```python
from build123d import *

# Parameters (mm, degrees)
F0_R     = 2.5
F1_DEPTH = 3
F2_R     = 1.5
F3_DEPTH = 10
F4_R     = 2.286


with BuildPart() as f1:
    # F0 (on Front) → F1 (new body)
    with BuildSketch(Plane.XZ):
        Circle(F0_R)
    extrude(amount=F1_DEPTH)

    # F2 (on face) → F3 (join)
    with BuildSketch(Plane(origin=(0, 0, 0), x_dir=(-1, 0, 0), z_dir=(0, 1, 0))):
        Circle(F2_R)
    extrude(amount=F3_DEPTH)

    # F4
    f4_edges = [f1.edges().sort_by_distance(p)[0] for p in [
        (-2.5, -3, 0),
    ]]
    fillet(f4_edges, radius=F4_R)


solid = f1.part
```
Input: part model. Units: mm. Frame: model coordinates. A direction names the side the tool comes from. Coordinates: 2 decimals unless noted, no trailing zeros. Write each loop counter-clockwise with the first axis right and the second up, starting at its lowest first coordinate (ties: lowest second). Pieces come first, ordered by that corner, then holes. Notation, with made-up numbers: M 80,11.25 L 106,11.25 A9 cw 106,28.25 Z; hole C 3,6 d2. An arc over 180 degrees is marked long. Use one line per item in the form item = value.
Q1. Material intervals for probe 1 along Z at (x, y) = (-0.1, -0.25); probe 2 along X at (y, z) = (1, -0.05), sorted ascending. Write a range as from..to.
Answer below:
probe_1 = -2.5..2.5
probe_2 = -1.5..1.5
Q2. Section A-A (y = 5). Return loops of the section in (x, z).
Answer below:
outline = C 0,0 d3
Q3. First-contact query: pin 1 (3 mm diameter, centred on y = 5.5, z = -1, fed in from +X); pin 2 (3 mm diameter, centred on y = 8.5, z = 1, fed in from -X). Flat tips, straight axial feed; report the tip coordinate or a pass-through.
Answer below:
pin_1 = 1.5
pin_2 = -1.5
Q4. Set-up query: faces 1 (the face through (0, 10, 0)), 2 (the face through (0, 0, -2)). Return all of +Z, -Z, +X, -X, +Y, -Y with unobstructed straight access to the full face (end or side cutting, diameter ignored); none if empty.
Answer below:
face_1 = +Z, -Z, +X, -X, +Y
face_2 = +Y
